from build123d import *

# Parameters (mm, degrees)
BOSS_EXTRUDE1_DEPTH = 15
SKETCH2_R           = 2.925
SKETCH2_R_2         = 3
CUT_EXTRUDE1_DEPTH  = 16
CUT_EXTRUDE2_DEPTH  = 5


with BuildPart() as part:
    # Sketch1 → Boss-Extrude1 (new body)
    with BuildSketch(Plane.XY):
        Polygon((7, -2.83), (22, 16), (17, 16), (0, -1), (-17, 16), (-22, 16), (-7, -2.83), (-7, -162.83), (7, -162.83), align=None)
    extrude(amount=BOSS_EXTRUDE1_DEPTH)

    # Sketch2 → Cut-Extrude1 (cut, through all)
    with BuildSketch(Plane.XY.offset(15)):
        with Locations((0, -132.83)):
            Circle(SKETCH2_R)
        with Locations((0, -152.83)):
            Circle(SKETCH2_R_2)
    extrude(amount=-CUT_EXTRUDE1_DEPTH, mode=Mode.SUBTRACT)

    # Sketch3 → Cut-Extrude2 (cut)
    with BuildSketch(Plane.XY.offset(15)):
        with BuildLine():
            Line((-7, -110.522582404), (-7, -162.83))
            Line((-7, -162.83), (7, -162.83))
            Line((7, -162.83), (7, -110.522582404))
            ThreePointArc((7, -110.522582404), (0, -115.33), (-7, -110.522582404))
        make_face()
    extrude(amount=-CUT_EXTRUDE2_DEPTH, mode=Mode.SUBTRACT)


solid = part.part
Design review of the part built by this model. Coordinates are the model's own, in mm. A direction names the side the tool comes from. Round coordinates to 2 decimals unless told otherwise and drop trailing zeros. Write each loop counter-clockwise with the first axis right and the second up, starting at its lowest first coordinate (ties: lowest second). Pieces come first, ordered by that corner, then holes.
Item 1: Consider section B-B on y = -152.83. Give the boundary of the cut face in (x, z).
Item 2: Consider section A-A on z = 3. Give the boundary of the cut face in (x, y) (3 decimals).
Item 3: For faces 4 (the flat face through (7, -84, 7)), 5 (the flat face through (-7, -82, 7)), 6 (the flat face through (9, 8, 7)), 7 (the flat face through (0, -73, 0)), 8 (the cylindrical face through (-0.38, -129.93, 5.07)), list the 3-axis set-ups (+Z, -Z, +X, -X, +Y, -Y) from which the entire face can be reached by the end or side of a thin tool; tool diameter is ignored.
Item 4: Consider section D-D on z = 13.25. Give the boundary of the cut face in (x, y), and give its area (3 significant figures).
Item 5: For pin 1 Ø4 at (x, z) = (-10, 4.5) entering from -Y; pin 2 Ø7.5 at (x, y) = (0, -132.83) entering from +Z; pin 3 Ø8 at (y, z) = (-87.5, 8) entering from -X, all flat-tipped, find the tip position at first contact; note any pin that passes through.
Item 6: Wall thickness on L1, parallel to Y at x = 0, z = 6 (3 decimals); L2, parallel to X at y = -132.83, z = 7 (3 decimals); L3, parallel to X at y = -152.83, z = 2.25: over which ranges is each line inside the solid? List them lowest first.
Item 7: Draft analysis for pull direction X (two halves, no side actions). For faces 1 (the cylindrical face through (0.13, -115.33, 12.54)), 2 (the cylindrical face through (1.384, -155.492, 5.07)), 3 (the flat face through (-14.605, 6.717, 7.395)), state which applies: released by +X, released by -X, zero draft, split by the parting line, or undercut.
Item 8: Consider section C-C on x = -4.5. Give the boundary of the cut face in (y, z), and give its area (3 significant figures).
Check values:
1. outline: (-7, 0) - (-3, 0) - (-3, 10) - (-7, 10) - close; (3, 0) - (7, 0) - (7, 10) - (3, 10) - close
2. outline: (-22, 16) - (-7, -2.83) - (-7, -162.83) - (7, -162.83) - (7, -2.83) - (22, 16) - (17, 16) - (0, -1) - (-17, 16) - close; hole circle Ø6 at (0, -152.83); hole circle Ø5.85 at (0, -132.83)
3. face 4: +Z, -Z, +X, -Y
3. face 5: +Z, -Z, -X, -Y
3. face 6: +Z, -Z, +Y
3. face 7: -Z, +X, -X, +Y, -Y
3. face 8: +Z, -Z
4. outline: (-22, 16) - (-7, -2.83) - (-7, -110.52) arc R7.5 ccw to (7, -110.52) - (7, -2.83) - (22, 16) - (17, 16) - (0, -1) - (-17, 16) - close
4. area: 1,810 mm2
5. pin 1: stops at y = -1.57
5. pin 2: stops at z = 10
5. pin 3: stops at x = -7
6. L1: y = -162.83 to -155.83, -149.83 to -135.755, -129.905 to -1
6. L2: x = -7 to -2.925, 2.925 to 7
6. L3: x = -7 to -3, 3 to 7
7. face 1: split by the parting line
7. face 2: undercut
7. face 3: released by -X
8. outline: (-162.83, 0) - (3.5, 0) - (3.5, 15) - (-113.83, 15) - (-113.83, 10) - (-162.83, 10) - close
8. area: 2,250 mm2
